from build123d import *

# Parameters (mm, degrees)
SKETCH1_W           = 38.1
SKETCH1_H           = 25.4
SKETCH1_R           = 1.65
BOSS_EXTRUDE1_DEPTH = 5
SKETCH2_R           = 3
CUT_EXTRUDE1_DEPTH  = 2.5
FILLET1_R           = 2


with BuildPart() as part:
    # Sketch1 → Boss-Extrude1 (new body)
    with BuildSketch(Plane(origin=(0, 0, 0), x_dir=(1, 0, 0), z_dir=(0, 1, 0))):
        with Locations((19.05, 12.7)):
            Rectangle(SKETCH1_W, SKETCH1_H)
        with Locations(Location((19.05, 5.16, 0), (0, 0, 270))):
            Circle(SKETCH1_R, mode=Mode.SUBTRACT)
        with Locations(Location((6, 19.4, 0), (0, 0, 270))):
            Circle(SKETCH1_R, mode=Mode.SUBTRACT)
        with Locations(Location((32.1, 19.4, 0), (0, 0, 90))):
            Circle(SKETCH1_R, mode=Mode.SUBTRACT)
    extrude(amount=BOSS_EXTRUDE1_DEPTH)

    # Sketch2 → Cut-Extrude1 (cut)
    with BuildSketch(Plane(origin=(0, 5, 0), x_dir=(1, 0, 0), z_dir=(0, 1, 0))):
        with Locations(Location((6, 19.4, 0), (0, 0, 270))):
            Circle(SKETCH2_R)
        with Locations(Location((19.05, 5.16, 0), (0, 0, 270))):
            Circle(SKETCH2_R)
        with Locations(Location((32.1, 19.4, 0), (0, 0, 270))):
            Circle(SKETCH2_R)
    extrude(amount=-CUT_EXTRUDE1_DEPTH, mode=Mode.SUBTRACT)

    # Fillet1
    fillet1_edges = [part.edges().sort_by_distance(p)[0] for p in [
        (38.1, 5, -12.7),
        (19.05, 5, -25.4),
        (0, 5, -12.7),
        (19.05, 5, 0),
    ]]
    fillet(fillet1_edges, radius=FILLET1_R)


solid = part.part
Verification items for the finished model (mm, model axes). A direction names the side the tool comes from. Coordinates: 2 decimals unless noted, no trailing zeros. Order: outer loops, then holes, each group sorted by start corner. A loop starts at its lowest first (then second) coordinate and runs counter-clockwise, first axis right, second up. Notation, with made-up numbers: M 36,52 L 77,52 A25 ccw 77,86 Z; hole C 27.25,-28 d7. An arc over 180 degrees is marked long. Return JSON: item names as keys, results as strings.
1) Cross-section at D-D, the plane x = 29.5. Record the boundary of the cut face in (y, z), and give its area (3 significant figures).
Answer list:
{"outline": "M 0,-25.4 L 3,-25.4 A2 ccw 5,-23.4 L 5,-20.9 L 2.5,-20.9 L 2.5,-17.9 L 5,-17.9 L 5,-2 A2 ccw 3,0 L 0,0 Z", "area": "118 mm2"}
2) Cross-section at B-B, the plane z = -5.16. Record the boundary of the cut face in (x, y).
Answer list:
{"outline": "M 0,0 L 17.4,0 L 17.4,2.5 L 16.05,2.5 L 16.05,5 L 2,5 A2 ccw 0,3 Z; M 20.7,0 L 38.1,0 L 38.1,3 A2 ccw 36.1,5 L 22.05,5 L 22.05,2.5 L 20.7,2.5 Z"}
3) Access from +Z, -Z, +X, -X, +Y, -Y to the whole of each face (thin tool, end or side, straight path). Record for faces 1 (the cylindrical face through (30.71, 1.23, -20.29)), 2 (the cylindrical face through (4.85, 3.77, -16.63)).
Answer list:
{"face 1": "+Y, -Y", "face 2": "+Y"}
4) Cross-section at C-C, the plane y = 4.2. Record the boundary of the cut face in (x, z), and give its area (3 significant figures).
Answer list:
{"outline": "M 0.4,-25 L 37.7,-25 L 37.7,-0.4 L 0.4,-0.4 Z; hole C 6,-19.4 d6; hole C 19.05,-5.16 d6; hole C 32.1,-19.4 d6", "area": "833 mm2"}
5) Gauge pin test, flat end, axial feed: pin 1 (1.8 mm diameter, centred on x = 20.5, z = -6, fed in from +Y). Record the tip position at first contact, or that the pin passes through.
Answer list:
{"pin 1": "y = 2.5"}
6) Thickness scan on L1, parallel to X at y = 3.2, z = -19.4; L2, parallel to X at y = 0.7, z = -19.4; L3, parallel to Z at x = 19.05, y = 1.65. Record the ranges inside material, lowest first. Write a range as [from, to].
Answer list:
{"L1": "[0.01, 3], [9, 29.1], [35.1, 38.09]", "L2": "[0, 4.35], [7.65, 30.45], [33.75, 38.1]", "L3": "[-25.4, -6.81], [-3.51, 0]"}
7) Cross-section at A-A, the plane x = 6. Record the boundary of the cut face in (y, z), and give its area (3 significant figures).
Answer list:
{"outline": "M 0,-25.4 L 3,-25.4 A2 ccw 5,-23.4 L 5,-22.4 L 2.5,-22.4 L 2.5,-21.05 L 0,-21.05 Z; M 0,-17.75 L 2.5,-17.75 L 2.5,-16.4 L 5,-16.4 L 5,-2 A2 ccw 3,0 L 0,0 Z", "area": "102 mm2"}
8) Release check for a two-part mould opening along X. For faces 3 (the cylindrical face through (20.44, 1.23, -4.27)), 4 (the cylindrical face through (37.5, 4.43, -12.88)), 5 (the flat face through (4.7, 2.5, -18.1)), 6 (the flat face through (0, 1, -13)) record: +X half, -X half, draft (parallel to the pull), parting line (faces both ways), or undercut.
Answer list:
{"face 3": "undercut", "face 4": "+X half", "face 5": "undercut", "face 6": "-X half"}
